Geometry check sheet. Reference: drawing and pictorial views, mm from the part's lowest x, y, z. A direction names the side the tool comes from. Coordinates: 2 decimals unless noted, no trailing zeros. Write each loop counter-clockwise with the first axis right and the second up, starting at its lowest first coordinate (ties: lowest second). Pieces come first, ordered by that corner, then holes. Notation, with made-up numbers: (-12, -33) -> (31, -33) arc R18 ccw to (31, -17) -> close; hole circle Ø1 at (-31, 8.25). An arc over 180 degrees is marked (long way). Use a Markdown table: item, result.
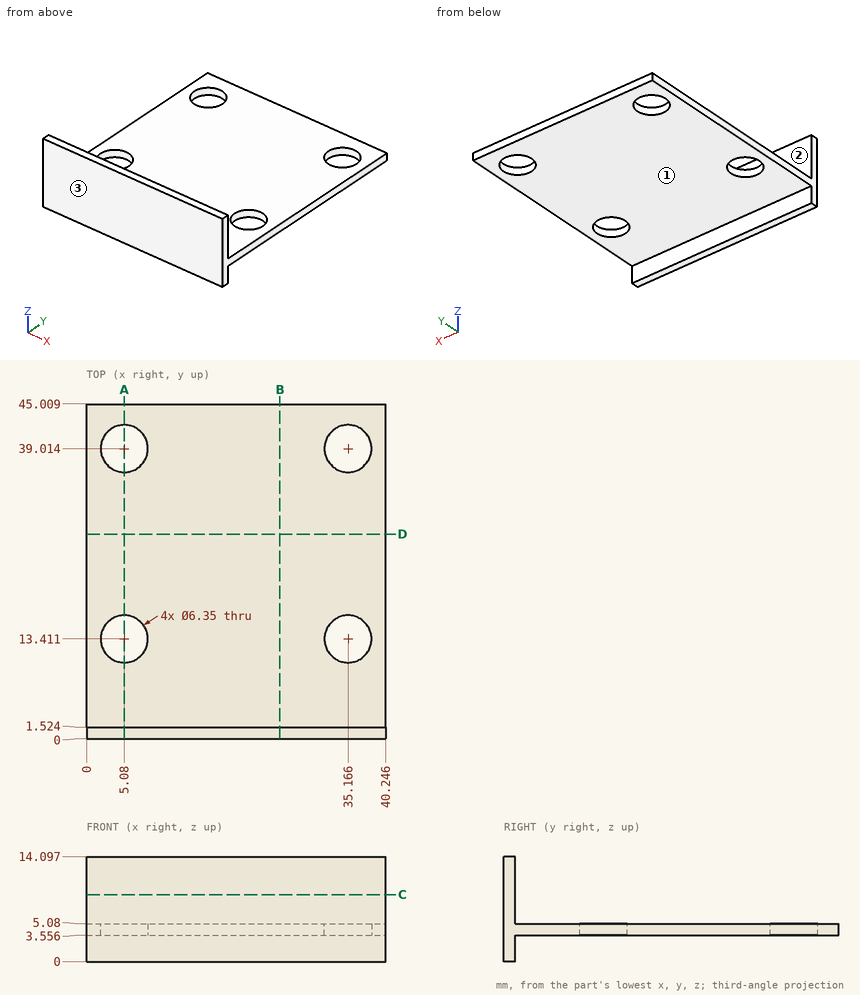
Item 1: Section check D-D on y = 27.5. Record the boundary of the cut face in (x, z).
Answer block:
| item | result |
|---|---|
| outline | (0, 3.56) -> (40.25, 3.56) -> (40.25, 5.08) -> (0, 5.08) -> close |
Item 2: Section check C-C on z = 9. Record the boundary of the cut face in (x, y).
Answer block:
| item | result |
|---|---|
| outline | (0, 0) -> (40.25, 0) -> (40.25, 1.52) -> (0, 1.52) -> close |
Item 3: Tool access check on the marked faces 1, 2 and 3. Record the directions out of +Z, -Z, +X, -X, +Y, -Y that give a thin tool (end or side, any length) a straight path to the whole face; none if there is none.
Answer block:
| item | result |
|---|---|
| face 1 | -Z, +X, -X, +Y |
| face 2 | +Z, +X, -X, +Y |
| face 3 | +Z, -Z, +X, -X, -Y |
Item 4: Section check A-A on x = 5.08. Record the boundary of the cut face in (y, z).
Answer block:
| item | result |
|---|---|
| outline | (0, 0) -> (1.52, 0) -> (1.52, 3.56) -> (10.24, 3.56) -> (10.24, 5.08) -> (1.52, 5.08) -> (1.52, 14.1) -> (0, 14.1) -> close; (16.59, 3.56) -> (35.84, 3.56) -> (35.84, 5.08) -> (16.59, 5.08) -> close; (42.19, 3.56) -> (45.01, 3.56) -> (45.01, 5.08) -> (42.19, 5.08) -> close |
Item 5: Section check B-B on x = 26. Record the boundary of the cut face in (y, z).
Answer block:
| item | result |
|---|---|
| outline | (0, 0) -> (1.52, 0) -> (1.52, 3.56) -> (45.01, 3.56) -> (45.01, 5.08) -> (1.52, 5.08) -> (1.52, 14.1) -> (0, 14.1) -> close |
Item 6: Depth check by flat-ended pin: P1, Ø5.5, axis at x = 35.17, y = 13.41, coming from the +Z side; P2, Ø8.5, axis at x = 35.17, y = 39.01, coming from the +Z side; P3, Ø5, axis at x = 25.5, y = 40, coming from the -Z side; P4, Ø3, axis at x = 28, z = 12.5, coming from the +Y side. Enter the tip coordinate at first touch or a pass-through.
Answer block:
| item | result |
|---|---|
| P1 | passes through |
| P2 | stops at z = 5.08 |
| P3 | stops at z = 3.56 |
| P4 | stops at y = 1.52 |
Item 7: Thickness scan on L1, parallel to Y at x = 5.08, z = 4.5; L2, parallel to Y at x = 29, z = 7.5; L3, parallel to Z at x = 30.5, y = 29. Record the ranges inside material, lowest first. Write a range as [from, to].
Answer block:
| item | result |
|---|---|
| L1 | y = [0, 10.24], [16.59, 35.84], [42.19, 45.01] |
| L2 | y = [0, 1.52] |
| L3 | z = [3.56, 5.08] |
